Geometry check sheet. Reference: the model listing, model coordinates, mm. Face numbers are marked on the shaded views. A direction names the side the tool comes from. Round coordinates to 2 decimals unless told otherwise and drop trailing zeros. Order: outer loops, then holes, each group sorted by start corner. A loop starts at its lowest first (then second) coordinate and runs counter-clockwise, first axis right, second up. Notation, with made-up numbers: (50.5, 26.5) - (89.5, 26.5) arc R20 cw to (89.5, 55.5) - close; hole circle Ø10 at (45, 21.5). An arc over 180 degrees is marked (long way). Return JSON: item names as keys, results as strings. Group by question number.
Q1. Sectioned sample at A-A, the plane x = 0. Record the cut outline in (y, z).
Q2. Gauge pin test, flat ends, axial feed: pin 1 Ø13.5 at (x, y) = (-56, -2) entering from -Z; pin 2 Ø8 at (x, z) = (86.5, -17.5) entering from +Y. Record the tip position at first contact, or that the pin passes through.
Q3. Sectioned sample at B-B, the plane y = 0. Record the cut outline in (x, z), then the cut area to 3 significant figures.
Q4. Sectioned sample at D-D, the plane x = -32. Record the cut outline in (y, z).
Q5. Material ranges on line 1 along Y through (x, z) = (0, -2.5); line 2 along Y through (x, z) = (136.5, -38); line 3 along Z through (x, y) = (132.5, 14.5), recorded low to high.
Q6. Sectioned sample at C-C, the plane z = 2. Record the cut outline in (x, y), then the cut area to 3 significant figures.
Q7. Tool access check on the marked faces 1 and 2. Record the directions out of +Z, -Z, +X, -X, +Y, -Y that give a thin tool (end or side, any length) a straight path to the whole face; none if there is none.
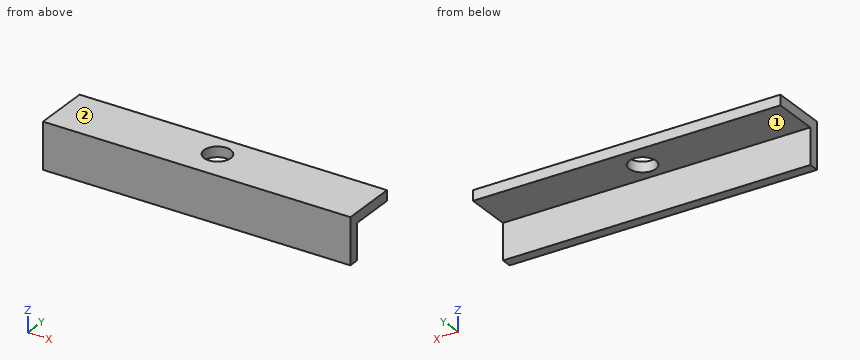
```python
from build123d import *

# Parameters (mm, degrees)
EXTRUDE_THIN1_DEPTH = 150
SKETCH2_R           = 13
CUT_EXTRUDE1_DEPTH  = 46


with BuildPart() as part:
    # Sketch1 → Extrude-Thin1 (new body, symmetric)
    with BuildSketch(Plane(origin=(0, 0, 0), x_dir=(0, 0, -1), z_dir=(1, 0, 0))):
        Polygon((-5, 23.80952381), (-5, -31.19047619), (40, -31.19047619), (40, -21.19047619), (5, -21.19047619), (5, 23.80952381), align=None)
    extrude(amount=EXTRUDE_THIN1_DEPTH, both=True)

    # Sketch2 → Cut-Extrude1 (cut, through all)
    with BuildSketch(Plane.XY.offset(5)):
        Circle(SKETCH2_R)
    extrude(amount=-CUT_EXTRUDE1_DEPTH, mode=Mode.SUBTRACT)


solid = part.part
```
Reply:
{
 "1": {"outline": "(-31.19, -40) - (-21.19, -40) - (-21.19, -5) - (-13, -5) - (-13, 5) - (-31.19, 5) - close; (13, -5) - (23.81, -5) - (23.81, 5) - (13, 5) - close"},
 "2": {"pin 1": "z = -5", "pin 2": "y = -21.19"},
 "3": {"outline": "(-150, -5) - (-13, -5) - (-13, 5) - (-150, 5) - close; (13, -5) - (150, -5) - (150, 5) - (13, 5) - close", "area": "2,740 mm^2"},
 "4": {"outline": "(-31.19, -40) - (-21.19, -40) - (-21.19, -5) - (23.81, -5) - (23.81, 5) - (-31.19, 5) - close"},
 "5": {"line 1": "-31.19 to -13, 13 to 23.81", "line 2": "-31.19 to -21.19", "line 3": "-5 to 5"},
 "6": {"outline": "(-150, -31.19) - (150, -31.19) - (150, 23.81) - (-150, 23.81) - close; hole circle Ø26 at (0, 0)", "area": "16,000 mm^2"},
 "7": {"face 1": "-Z, +X, -X, +Y", "face 2": "+Z, +X, -X, +Y, -Y"}
}
